The model under review builds one solid part; all positions refer to its coordinate system, in mm. Face numbers are marked on the shaded views. A direction names the side the tool comes from. Round coordinates to 2 decimals unless told otherwise and drop trailing zeros. Order: outer loops, then holes, each group sorted by start corner. A loop starts at its lowest first (then second) coordinate and runs counter-clockwise, first axis right, second up.
1) Consider section B-B (z = 24.5). Give the boundary of the cut face in (x, y).
2) Consider section A-A (y = 0). Give the boundary of the cut face in (x, z), then the cut area to 3 significant figures.
3) Mouldability with a two-part tool opening along X and no side actions: class the marked faces 3, 4 and 5 as pulls with the +X half, pulls with the -X half, needs draft (parallel to the pull), parting line crosses it, or undercut.
4) Clearance check with flat-ended pins moving along their axes: P1, Ø2, axis at x = 26.5, z = -44, coming from the -Y side; P2, Ø10, axis at x = -20.5, z = -32.5, coming from the -Y side; P3, Ø12, axis at x = 24, z = -26.5, coming from the -Y side. State where each tip first meets the part, or that it passes through.
5) To check wall thickness, follow L1, parallel to X at y = 48.5, z = 36.5; L2, parallel to Z at x = -42, y = 0. State the ranges of each line that lie inside material, in increasing order.
6) Consider section C-C (z = -19). Give the boundary of the cut face in (x, y), then the cut area to 3 significant figures.
7) Machinability: for the marked faces 1 and 2, which of the approach directions +Z, -Z, +X, -X, +Y, -Y give a long, thin tool a straight path to every point of the face, cutting with its end or side? Answer none if there is none.
8) Consider section D-D (y = 41.5). Give the boundary of the cut face in (x, z).
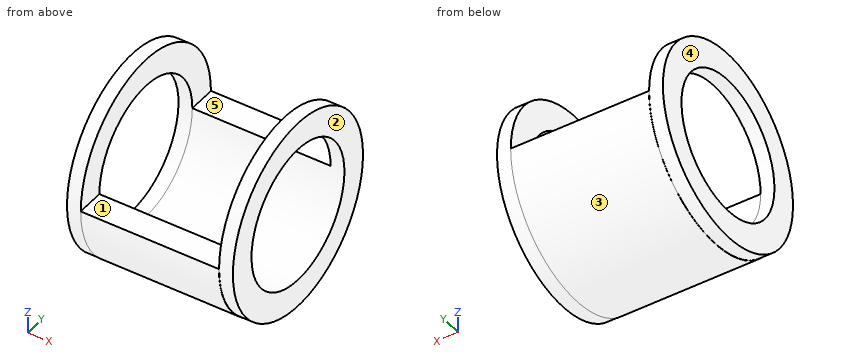
from build123d import *

# Parameters (mm, degrees)
ESQUISSE1_W                  = 10
ESQUISSE1_H                  = 70
ESQUISSE1_4_W                = 10
ESQUISSE1_4_H                = 70
ESQUISSE14_W                 = 100
ESQUISSE14_H                 = 70.182088946
R_VOLUTION5_ANGLE            = 180
ESQUISSE15_R                 = 50
ENL_V_MAT_EXTRU_1_DEPTH      = 111
ENL_V_MAT_EXTRU_1_DEPTH_BACK = 11


with BuildPart() as part:
    # Esquisse1 → R_vol.-Mince2 (revolve)
    with BuildSketch(Plane.XY):
        with Locations((-45, 35)):
            Rectangle(ESQUISSE1_W, ESQUISSE1_H)
    revolve(axis=Axis((-50, 0, 0), (1, 0, 0)))



with BuildPart() as body_2:
    # Esquisse1_4 → R_vol.-Mince3 (revolve)
    with BuildSketch(Plane.XY):
        with Locations((65, 35)):
            Rectangle(ESQUISSE1_4_W, ESQUISSE1_4_H)
    revolve(axis=Axis((-50, 0, 0), (1, 0, 0)))


with BuildPart() as part_1:
    add(part.part)

    add(body_2.part)  # R_volution5 merges body 2
    # Esquisse14 → R_volution5 (revolve)
    with BuildSketch(Plane.XY):
        with Locations((10, 35.091044473)):
            Rectangle(ESQUISSE14_W, ESQUISSE14_H)
    revolve(axis=Axis((60, 0, 0), (-1, 0, 0)), revolution_arc=R_VOLUTION5_ANGLE)

    # Esquisse15 → Enl_v. mat.-Extru.1 (cut, two sides)
    with BuildSketch(Plane(origin=(-40, 0, 0), x_dir=(0, 0, -1), z_dir=(1, 0, 0))) as enl_v_mat_extru_1_sk:
        Circle(ESQUISSE15_R)
    extrude(amount=ENL_V_MAT_EXTRU_1_DEPTH, mode=Mode.SUBTRACT)
    extrude(enl_v_mat_extru_1_sk.sketch, amount=-ENL_V_MAT_EXTRU_1_DEPTH_BACK, mode=Mode.SUBTRACT)


solid = part_1.part
Answer below:
1. outline: (-50, -65.57) - (-40, -65.57) - (-40, -43.59) - (-50, -43.59) - close; (-50, 43.59) - (-40, 43.59) - (-40, 65.57) - (-50, 65.57) - close; (60, -65.57) - (70, -65.57) - (70, -43.59) - (60, -43.59) - close; (60, 43.59) - (70, 43.59) - (70, 65.57) - (60, 65.57) - close
2. outline: (-50, -70) - (-40, -70) - (-40, -70.18) - (60, -70.18) - (60, -70) - (70, -70) - (70, -50) - (-50, -50) - close; (-50, 50) - (-40, 50) - (-40, 70) - (-50, 70) - close; (60, 50) - (70, 50) - (70, 70) - (60, 70) - close
2. area: 2,820 mm2
3. face 3: needs draft
3. face 4: pulls with the -X half
3. face 5: undercut
4. P1: stops at y = -55.47
4. P2: stops at y = -64.57
4. P3: stops at y = -67.12
5. L1: x = -50 to -40, 60 to 70
5. L2: z = -70 to -50, 50 to 70
6. outline: (-50, -67.37) - (-40, -67.37) - (-40, -67.56) - (60, -67.56) - (60, -67.37) - (70, -67.37) - (70, -46.25) - (-50, -46.25) - close; (-50, 46.25) - (70, 46.25) - (70, 67.37) - (60, 67.37) - (60, 67.56) - (-40, 67.56) - (-40, 67.37) - (-50, 67.37) - close
6. area: 5,110 mm2
7. face 1: +Z, +Y, -Y
7. face 2: +Z, -Z, +X, +Y, -Y
8. outline: (-50, -56.37) - (-40, -56.37) - (-40, -56.6) - (60, -56.6) - (60, -56.37) - (70, -56.37) - (70, -27.89) - (-50, -27.89) - close; (-50, 27.89) - (-40, 27.89) - (-40, 56.37) - (-50, 56.37) - close; (60, 27.89) - (70, 27.89) - (70, 56.37) - (60, 56.37) - close
